Verification items for the finished model (mm, model axes). Round coordinates to 2 decimals unless told otherwise and drop trailing zeros. Write each loop counter-clockwise with the first axis right and the second up, starting at its lowest first coordinate (ties: lowest second). Pieces come first, ordered by that corner, then holes.
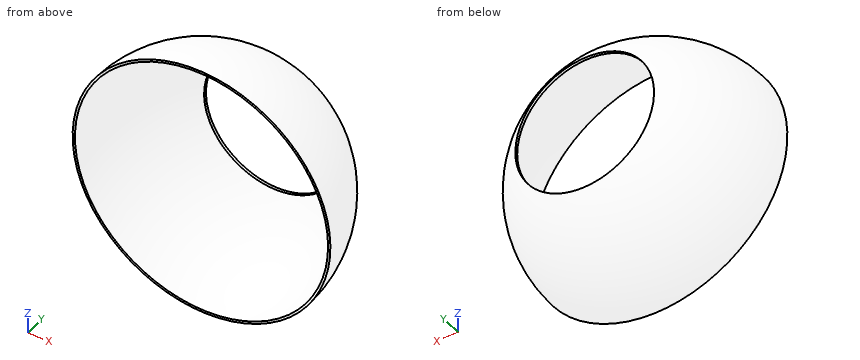
Autodesk Inventor part; units mm, degrees
ref_plane "Work Plane2" through (0, 0, 0) normal (-0.7071068, 0, 0.7071068) x (0, 1, 0)
ref_plane "Work Plane3" through (0, 1, 0) normal (0, -1, 0) x (1, 0, 0)
ref_plane "YZ Plane" through (0, 0, 0) normal (1, 0, 0) x (0, 1, 0)
sketch "Sketch1" plane through (0, 0, 0) normal (0, 1, 0) x (-1, 0, 0)
  line L0 (0, 0) -> (25, 0)
  line L1 (25, 0) -> (25, -25)
  line L2 (25, -25) -> (0, -25)
  line L3 (0, -25) -> (0, 0)
  circle A0 centre (12.5, -12.5) radius 17.6777
  circle A1 centre (12.5, -12.5) radius 21.86
  dimension "d0" = 25
  dimension "d1" = 25
  dimension "d2" = 43.72
extrude "Extrusion1" add sketch "Sketch1" along normal blind 1 contours L0 L1 L2 L3
ref_plane "Work Plane2" through (0, 0, 0) normal (-0.7071068, 0, 0.7071068) x (0, 1, 0)
sketch "Sketch3" plane through (0, 0, 0) normal (-0.7071068, 0, 0.7071068) x (0, 1, 0)
  line L0 (1, 0) -> (1, 17.6777)
  line L1 (1, 17.6777) -> (1, 35.3553)
  line L2 (1, 17.6777) -> (7.5, 17.6777) construction
  arc A0 (1, 0) -> (1, 35.3553) centre (-19.7885, 17.6777) ccw construction
  circle A1 centre (-19.7885, 17.6777) radius 27.375 construction
  circle A2 centre (-19.7885, 17.6777) radius 27.375
  circle A3 centre (-19.7885, 17.6777) radius 27.875
  line L3 (7.5, 17.6777) -> (8.0865, 17.6777)
  line L4 (-19.7885, 45.0527) -> (-19.7885, 45.5527)
  line L5 (-19.7885, 17.6777) -> (-5.3263, 17.6777)
  line L6 (-19.7885, 17.6777) -> (-19.7885, 45.0527)
  point P0 (0, 0)
  point P1 (7.5865, 17.6777)
  dimension "d10" = 6.5
  dimension "d11" = 54.75
  dimension "d12" = 55.75
revolve "Revolution1" add sketch "Sketch3" angle 360 about axis through (-12.5, -19.7885, -12.5) along (0, 1, 0) picked at (-9.7302, 43.3292) contours A2 L4 A3 L3
ref_plane "Work Plane3" through (0, 1, 0) normal (0, -1, 0) x (1, 0, 0)
sketch "Sketch5" plane through (0, 0, 0) normal (0, -1, 0) x (1, 0, 0)
  line L0 (0, -25) -> (-25, -25) construction
  line L1 (0, 0) -> (0, -25) construction
  line L2 (-25, 0) -> (0, 0) construction
  line L3 (-25, -25) -> (-25, 0) construction
  line L4 (-12.5, 0) -> (-12.5, -12.5) construction
  circle A0 centre (-12.5, -12.5) radius 15
  dimension "d33" = 12.5
  dimension "d34" = 30
extrude "Extrusion3" cut sketch "Sketch5" against normal blind 10
sketch "Sketch6" plane through (0, 0, 0) normal (0, -1, 0) x (1, 0, 0)
  arc A0 (-25, -20.7916) -> (-20.7916, -25) centre (-12.5, -12.5) ccw
  line L0 (0, -25) -> (-4.2084, -25)
  line L1 (0, 0) -> (0, -4.2084)
  line L2 (-25, 0) -> (-20.7916, 0)
  line L3 (-25, -25) -> (-25, -20.7916)
  line L4 (-20.7916, -25) -> (-25, -25)
  arc A1 (-4.2084, -25) -> (0, -20.7916) centre (-12.5, -12.5) ccw
  line L5 (0, -20.7916) -> (0, -25)
  arc A2 (0, -4.2084) -> (-4.2084, 0) centre (-12.5, -12.5) ccw
  line L6 (-4.2084, 0) -> (0, 0)
  arc A3 (-20.7916, 0) -> (-25, -4.2084) centre (-12.5, -12.5) ccw
  line L7 (-25, -4.2084) -> (-25, 0)
extrude "Extrusion4" cut sketch "Sketch6" against normal blind 1
properties part number "Ball"
Q1. Material ranges on line 1 along Z through (x, y) = (-12.5, 3.4); line 2 along X through (y, z) = (3.3, -12.5); line 3 along X through (y, z) = (-17.25, 7), recorded low to high.
Recorded:
line 1: z = -27.97 to -27.5, 2.5 to 2.97
line 2: x = -28.12 to -27.5, 2.5 to 3.12
line 3: x = -32.26 to -31.54, 6.54 to 7.26
Q2. Sectioned sample at D-D (x = -34). Enter the section's corners in (y, z), plus the area to 3 significant figures.
Recorded:
outline: (-19.79, -30.24) arc R17.74 ccw to (-19.79, 5.24) - (-19.79, 4.45) arc R16.95 cw to (-19.79, -29.45) - close
area: 43.4 mm2
Q3. Sectioned sample at C-C (y = -3.25). Enter the section's corners in (x, z).
Recorded:
outline: circle Ø44.88 at (-12.5, -12.5); hole circle Ø43.63 at (-12.5, -12.5)
Q4. Depth check by flat-ended pin: P1, Ø5, axis at x = -10, y = -11, coming from the +Z side; P2, Ø2, axis at x = 7, z = -0.5, coming from the +Y side; P3, Ø5, axis at x = -30, z = -9, coming from the -Y side. Enter the tip coordinate at first touch or a pass-through.
Recorded:
P1: stops at z = 14.57
P2: stops at y = -2.54
P3: stops at y = -1.47
Q5. Sectioned sample at A-A (x = -8). Enter the section's corners in (y, z).
Recorded:
outline: (-19.79, -40.01) arc R27.51 ccw to (3.71, -26.81) - (3.11, -26.81) arc R27 cw to (-19.79, -39.5) - close; (-19.79, 14.5) arc R27 cw to (3.11, 1.81) - (3.71, 1.81) arc R27.51 ccw to (-19.79, 15.01) - close
